from build123d import *

# Parameters (mm, degrees)
SKETCH1_W           = 88
SKETCH1_H           = 88
BOSS_EXTRUDE1_DEPTH = 4
SKETCH2_W           = 41.655
SKETCH2_H           = 88
SKETCH2_W_2         = 33.655
SKETCH2_H_2         = 82.55
BOSS_EXTRUDE2_DEPTH = 28.575
SKETCH4_W           = 33.655
SKETCH4_H           = 82.55
CUT_EXTRUDE1_DEPTH  = 69.472845895
SKETCH5_W           = 41.655
SKETCH5_H           = 88
BOSS_EXTRUDE3_DEPTH = 4
SKETCH6_R           = 13.97
CUT_EXTRUDE2_DEPTH  = 3.175
SKETCH7_R           = 12.7
CUT_EXTRUDE3_DEPTH  = 71.622659253
SKETCH8_W           = 60
SKETCH8_H           = 30
CUT_EXTRUDE4_DEPTH  = 4
SKETCH9_W           = 8.7752
SKETCH9_H           = 8.7752
SKETCH9_W_2         = 4.7752
SKETCH9_H_2         = 4.7752
BOSS_EXTRUDE4_DEPTH = 5.6764
SKETCH10_R          = 1.1
CUT_EXTRUDE5_DEPTH  = 73.17846372
SKETCH11_R          = 1.1
CUT_EXTRUDE6_DEPTH  = 71.236248654
BOSS_EXTRUDE5_DEPTH = 30
CUT_EXTRUDE7_DEPTH  = 27.5


with BuildPart() as part:
    # Sketch1 → Boss-Extrude1 (new body)
    with BuildSketch(Plane(origin=(0, 0, 0), x_dir=(1, 0, 0), z_dir=(0, 1, 0))):
        Rectangle(SKETCH1_W, SKETCH1_H)
    extrude(amount=BOSS_EXTRUDE1_DEPTH)

    # Sketch2 → Boss-Extrude2 (add)
    with BuildSketch(Plane(origin=(0, 4, 0), x_dir=(1, 0, 0), z_dir=(0, 1, 0))):
        Rectangle(SKETCH2_W, SKETCH2_H)
        Rectangle(SKETCH2_W_2, SKETCH2_H_2, mode=Mode.SUBTRACT)
    extrude(amount=BOSS_EXTRUDE2_DEPTH)

    # Sketch4 → Cut-Extrude1 (cut, through all)
    with BuildSketch(Plane(origin=(0, 4, 0), x_dir=(1, 0, 0), z_dir=(0, 1, 0))):
        Rectangle(SKETCH4_W, SKETCH4_H)
    extrude(amount=-CUT_EXTRUDE1_DEPTH, mode=Mode.SUBTRACT)

    # Sketch5 → Boss-Extrude3 (add)
    with BuildSketch(Plane(origin=(0, 32.575, 0), x_dir=(1, 0, 0), z_dir=(0, 1, 0))):
        Rectangle(SKETCH5_W, SKETCH5_H)
    extrude(amount=BOSS_EXTRUDE3_DEPTH)

    # Sketch6 → Cut-Extrude2 (cut)
    with BuildSketch(Plane(origin=(0, 36.575, 0), x_dir=(1, 0, 0), z_dir=(0, 1, 0))):
        with Locations(Location((0, 0, 0), (0, 0, 270))):
            Circle(SKETCH6_R)
    extrude(amount=-CUT_EXTRUDE2_DEPTH, mode=Mode.SUBTRACT)

    # Sketch7 → Cut-Extrude3 (cut, through all)
    with BuildSketch(Plane(origin=(0, 33.4, 0), x_dir=(1, 0, 0), z_dir=(0, 1, 0))):
        with Locations(Location((0, 0, 0), (0, 0, 270))):
            Circle(SKETCH7_R)
    extrude(amount=-CUT_EXTRUDE3_DEPTH, mode=Mode.SUBTRACT)

    # Sketch8 → Cut-Extrude4 (cut)
    with BuildSketch(Plane.XZ):
        Rectangle(SKETCH8_W, SKETCH8_H)
    extrude(amount=-CUT_EXTRUDE4_DEPTH, mode=Mode.SUBTRACT)

    # Sketch9 → Boss-Extrude4 (add)
    # profile 1 of 4: a face of its own
    with BuildSketch(Plane.XZ):
        with Locations((-25.6124, 19.3876)):
            Rectangle(SKETCH9_W, SKETCH9_H)
        with Locations((-25.6124, 19.3876)):
            Rectangle(SKETCH9_W_2, SKETCH9_H_2, mode=Mode.SUBTRACT)
    # profile 2 of 4: a face of its own
    with BuildSketch(Plane.XZ):
        with Locations((25.6124, 19.3876)):
            Rectangle(SKETCH9_W, SKETCH9_H)
        with Locations((25.6124, 19.3876)):
            Rectangle(SKETCH9_W_2, SKETCH9_H_2, mode=Mode.SUBTRACT)
    # profile 3 of 4: a face of its own
    with BuildSketch(Plane.XZ):
        with Locations((25.6124, -19.3876)):
            Rectangle(SKETCH9_W, SKETCH9_H)
        with Locations((25.6124, -19.3876)):
            Rectangle(SKETCH9_W_2, SKETCH9_H_2, mode=Mode.SUBTRACT)
    # profile 4 of 4: a face of its own
    with BuildSketch(Plane.XZ):
        with Locations((-25.6124, -19.3876)):
            Rectangle(SKETCH9_W, SKETCH9_H)
        with Locations((-25.6124, -19.3876)):
            Rectangle(SKETCH9_W_2, SKETCH9_H_2, mode=Mode.SUBTRACT)
    extrude(amount=-BOSS_EXTRUDE4_DEPTH)

    # Sketch10 → Cut-Extrude5 (cut, through all)
    with BuildSketch(Plane.XZ):
        with Locations(Location((-25.6124, 19.3876, 0), (0, 0, 270))):
            Circle(SKETCH10_R)
        with Locations(Location((25.6124, 19.3876, 0), (0, 0, 270))):
            Circle(SKETCH10_R)
        with Locations(Location((25.6124, -19.3876, 0), (0, 0, 270))):
            Circle(SKETCH10_R)
        with Locations(Location((-25.6124, -19.3876, 0), (0, 0, 270))):
            Circle(SKETCH10_R)
    extrude(amount=-CUT_EXTRUDE5_DEPTH, mode=Mode.SUBTRACT)

    # Sketch11 → Cut-Extrude6 (cut, through all)
    with BuildSketch(Plane(origin=(0, 4, 0), x_dir=(1, 0, 0), z_dir=(0, 1, 0))):
        with Locations(Location((-38.6124, 39.6124, 0), (0, 0, 270))):
            Circle(SKETCH11_R)
        with Locations(Location((38.6124, 39.6124, 0), (0, 0, 90))):
            Circle(SKETCH11_R)
        with Locations(Location((38.6124, -39.6124, 0), (0, 0, 270))):
            Circle(SKETCH11_R)
        with Locations(Location((-38.6124, -39.6124, 0), (0, 0, 90))):
            Circle(SKETCH11_R)
    extrude(amount=-CUT_EXTRUDE6_DEPTH, mode=Mode.SUBTRACT)

    # Sketch14 → Boss-Extrude5 (add, symmetric)
    with BuildSketch(Plane(origin=(0, 0, 0), x_dir=(0, 0, -1), z_dir=(1, 0, 0))):
        Polygon((-44, 4), (-48.238152403, 4), (-52.828513848, 0), (-44, 0), align=None)
        Polygon((44, 0), (44, 4), (48.238152403, 4), (52.828513848, 0), align=None)
    extrude(amount=BOSS_EXTRUDE5_DEPTH, both=True)

    # Sketch15 → Cut-Extrude7 (cut, symmetric)
    with BuildSketch(Plane(origin=(0, 0, 0), x_dir=(0, 0, -1), z_dir=(1, 0, 0))):
        Polygon((-50.081518623, 2.393707125), (-47.995663595, 0), (-50.74265882, -2.393707125), (-52.828513848, 0), align=None)
        Polygon((52.828513848, 0), (50.081518623, 2.393707125), (47.995663595, 0), (50.74265882, -2.393707125), align=None)
    extrude(amount=CUT_EXTRUDE7_DEPTH, both=True, mode=Mode.SUBTRACT)


solid = part.part
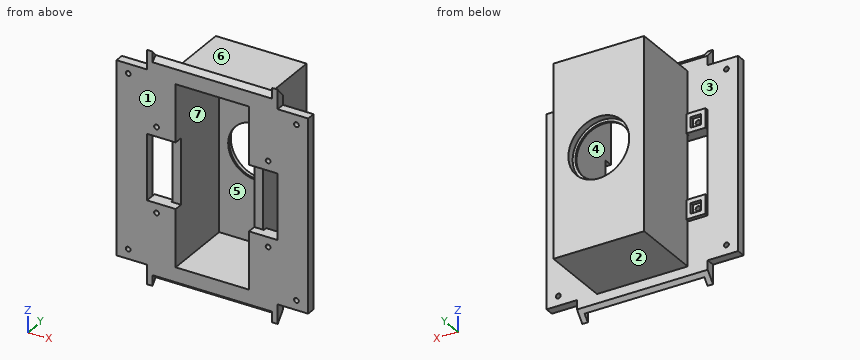
Can you work these out from the model? Positions are in its coordinate system, mm. Face numbers are marked on the shaded views. A direction names the side the tool comes from. Give positions to 0.01 mm unless a question says otherwise; leave off trailing zeros. Loops run counter-clockwise (first coordinate to the right, second up) from the corner with the lowest first, then second, coordinate; pieces in that order, holes last. Notation, with made-up numbers: (88.5, -40) - (108.5, -40) arc R21 cw to (108.5, -32) - close; hole circle Ø3 at (45.25, 62.5). An arc over 180 degrees is marked (long way). Return JSON: item names as keys, results as strings.
1. I want a section at A-A on z = 0. Please give me the cut outline in (x, y) (1 decimal).
Output values:
{"outline": "(-44, 0) - (-30, 0) - (-30, 4) - (-44, 4) - close; (-20.8, 4) - (-16.8, 4) - (-16.8, 32.6) - (-12.7, 32.6) - (-12.7, 33.4) - (-14, 33.4) - (-14, 36.6) - (-20.8, 36.6) - close; (12.7, 32.6) - (16.8, 32.6) - (16.8, 4) - (20.8, 4) - (20.8, 36.6) - (14, 36.6) - (14, 33.4) - (12.7, 33.4) - close; (30, 0) - (44, 0) - (44, 4) - (30, 4) - close"}
2. I want a section at B-B on y = 31. Please give me the cut outline in (x, z) (1 decimal), and give its area (3 significant figures).
Output values:
{"outline": "(-20.8, -44) - (20.8, -44) - (20.8, 44) - (-20.8, 44) - close; hole (-16.8, -41.3) - (16.8, -41.3) - (16.8, 41.3) - (-16.8, 41.3) - close", "area": "887 mm²"}
3. I'm going to push flat-ended pins straight in: pin 1 Ø0.5 at (y, z) = (4.5, 20.5) entering from +X; pin 2 Ø2 at (y, z) = (19.5, -36.5) entering from -X; pin 3 Ø3.5 at (x, z) = (25.61, -19.39) entering from +Y; pin 4 Ø8 at (x, z) = (25, -5.5) entering from +Y. Where does each tip first touch, or does it pass through?
Output values:
{"pin 1": "stops at x = 30", "pin 2": "stops at x = -20.83", "pin 3": "stops at y = 4", "pin 4": "passes through"}
4. We'd pull the mould along X, two halves only. Please class the marked faces 5, 6 and 7: +X half, -X half, draft (parallel to the pull), parting line (faces both ways), or undercut.
Output values:
{"face 5": "undercut", "face 6": "draft", "face 7": "undercut"}
5. I want a section at C-C on x = 0. Please give me the cut outline in (y, z) (3 decimals), and give its area (3 significant figures).
Output values:
{"outline": "(0, -47.996) - (2.394, -50.082) - (4, -48.238) - (4, -44) - (36.575, -44) - (36.575, -13.97) - (33.4, -13.97) - (33.4, -12.7) - (32.575, -12.7) - (32.575, -41.275) - (0, -41.275) - close; (0, 41.275) - (32.575, 41.275) - (32.575, 12.7) - (33.4, 12.7) - (33.4, 13.97) - (36.575, 13.97) - (36.575, 44) - (4, 44) - (4, 48.238) - (2.394, 50.082) - (0, 47.996) - close", "area": "461 mm²"}
6. If I drill on line 1 (X direction, y = 23, z = -5); line 2 (X direction, y = 32.95, z = 0); line 3 (Z direction, x = -6.5, y = 19) (3 decimals), over which ranges is the centre line in solid material (lowest first)?
Output values:
{"line 1": "x = -20.83 to -16.83, 16.83 to 20.83", "line 2": "x = -20.83 to -12.7, 12.7 to 20.83", "line 3": "z = -44 to -41.275, 41.275 to 44"}
7. For the marked faces 1, 2, 3 and 4, which set-ups out of +Z, -Z, +X, -X, +Y, -Y let a thin tool reach every point of the face, with its end or its side?
Output values:
{"face 1": "+Z, -Z, +X, -X, -Y", "face 2": "-Z, +X, -X, +Y", "face 3": "+Y", "face 4": "-Y"}
